Design review of the part built by this model. Coordinates are the model's own, in mm. Face numbers are marked on the shaded views. Coordinates: 2 decimals unless noted, no trailing zeros. Loops run counter-clockwise (first coordinate to the right, second up) from the corner with the lowest first, then second, coordinate; pieces in that order, holes last. Notation, with made-up numbers: (-25, 36.25) -> (-6, 36.25) arc R30 cw to (-6, 67.25) -> close; hole circle Ø6 at (20, 6). An arc over 180 degrees is marked (long way). Use CSV: the item, a comma, the result in double quotes.
```python
from build123d import *

# Parameters (mm, degrees)
PAD025_DEPTH         = 3
POCKET010_DEPTH      = 1.5
SKETCH059_W          = 32.687891
SKETCH059_H          = 10.975497
POCKET015_DEPTH      = 20.001
POCKET015_DEPTH_BACK = 15.001
FILLET006_R          = 1


with BuildPart() as part:
    # Sketch049 → Pad025 (new body)
    with BuildSketch(Plane.XY):
        with BuildLine():
            Line((-13, 15), (-5, 15))
            ThreePointArc((5, 15), (0, 20), (-5, 15))
            Line((5, 15), (13, 15))
            Line((13, 15), (13, -15))
            Line((13, -15), (-13, -15))
            Line((-13, -15), (-13, 15))
        make_face()
    extrude(amount=-PAD025_DEPTH)

    # Sketch050 → Pocket010 (cut)
    with BuildSketch(Plane.XY):
        with BuildLine():
            ThreePointArc((7.25, 0), (0, 7.25), (-7.25, 0))
            Line((-7.25, 0), (-7.25, -12.1))
            Line((-7.25, -12.1), (7.25, -12.1))
            Line((7.25, -12.1), (7.25, 0))
        make_face()
    extrude(amount=-POCKET010_DEPTH, mode=Mode.SUBTRACT)

    # Sketch059 → Pocket015 (cut, two sides)
    with BuildSketch(Plane.XZ) as pocket015_sk:
        with Locations((-0.0886585, -1.0893715)):
            Rectangle(SKETCH059_W, SKETCH059_H)
        with BuildLine():
            Line((10, 0), (-10, 0))
            Line((-10, 0), (-11.2928932188, -1.2928932188))
            ThreePointArc((-11.2928932188, -1.2928932188), (-11.5096659701, -2.3826834324), (-10.5857864376, -3))
            Line((-10.5857864376, -3), (10.5857864376, -3))
            ThreePointArc((10.5857864376, -3), (11.5096659701, -2.3826834324), (11.2928932188, -1.2928932188))
            Line((11.2928932188, -1.2928932188), (10, 0))
        make_face(mode=Mode.SUBTRACT)
    extrude(amount=-POCKET015_DEPTH, mode=Mode.SUBTRACT)
    extrude(pocket015_sk.sketch, amount=POCKET015_DEPTH_BACK, mode=Mode.SUBTRACT)

    # Fillet006
    fillet006_edges = [part.edges().sort_by_distance(p)[0] for p in [
        (0, -15, -3),
        (0, 20, -3),
        (7.792893, 15, -3),
        (-7.792893, 15, -3),
    ]]
    fillet(fillet006_edges, radius=FILLET006_R)


with BuildPart() as part_1:
    # Body017 placement: moved
    add(part.part.moved(Location((0, 0, -0.2))))


solid = part_1.part
```
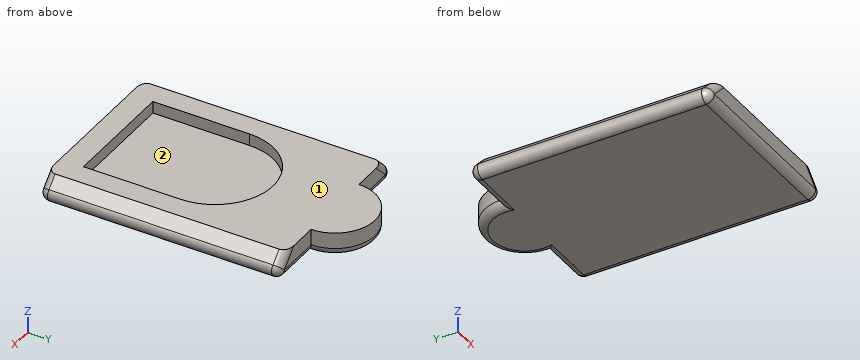
Item 1: Add section A-A (y = -1.5). Give the boundary of the cut face in (x, z), then the cut area to 3 significant figures.
Checked values:
outline,"(-11.29, -1.49) arc R1 ccw to (-10.59, -3.2) -> (10.59, -3.2) arc R1 ccw to (11.29, -1.49) -> (10, -0.2) -> (7.25, -0.2) -> (7.25, -1.7) -> (-7.25, -1.7) -> (-7.25, -0.2) -> (-10, -0.2) -> close"
area,"44.8 mm^2"
Item 2: To check wall thickness, follow line 1 along X through (y, z) = (-2, -2.9); line 2 along Z through (x, y) = (4.25, -5); line 3 along Y through (x, z) = (-1, -1.25). State the ranges of each line that lie inside material, in increasing order.
Checked values:
line 1,"-11.3 to 11.3"
line 2,"-3.2 to -1.7"
line 3,"-15 to -12.1, 7.18 to 19.9"
Item 3: Add section B-B (x = 0). Give the boundary of the cut face in (y, z), then the cut area to 3 significant figures.
Checked values:
outline,"(-15, -2.2) arc R1 ccw to (-14, -3.2) -> (19, -3.2) arc R1 ccw to (20, -2.2) -> (20, -0.2) -> (7.25, -0.2) -> (7.25, -1.7) -> (-12.1, -1.7) -> (-12.1, -0.2) -> (-15, -0.2) -> close"
area,"75.5 mm^2"
Item 4: Add section D-D (y = 9.5). Give the boundary of the cut face in (x, z), then the cut area to 3 significant figures.
Checked values:
outline,"(-11.29, -1.49) arc R1 ccw to (-10.59, -3.2) -> (10.59, -3.2) arc R1 ccw to (11.29, -1.49) -> (10, -0.2) -> (-10, -0.2) -> close"
area,"66.5 mm^2"
Item 5: Draft analysis for pull direction Y (two halves, no side actions). For the marked faces 1 and 2, state which applies: pulls with the +Y half, pulls with the -Y half, needs draft (parallel to the pull), parting line crosses it, or undercut.
Checked values:
face 1,"needs draft"
face 2,"undercut"
Item 6: Add section C-C (x = -7.75). Give the boundary of the cut face in (y, z), then the cut area to 3 significant figures.
Checked values:
outline,"(-15, -2.2) arc R1 ccw to (-14, -3.2) -> (14, -3.2) arc R1 ccw to (15, -2.2) -> (15, -0.2) -> (-15, -0.2) -> close"
area,"89.6 mm^2"
Item 7: Clearance check with flat-ended pins moving along their axes: pin 1 (0.6 mm diameter, centred on x = -6.5, z = -1, fed in from +Y); pin 2 (1.6 mm diameter, centred on y = -7, z = -1, fed in from +X); pin 3 (0.8 mm diameter, centred on y = -5.5, z = -1.5, fed in from -X). State where each tip first meets the part, or that it passes through.
Checked values:
pin 1,"y = 15"
pin 2,"x = 11.5"
pin 3,"x = -11.54"
